Check sheet for the drawn part. Datum: minimum x, y, z corner. Units: mm. Give positions to 0.01 mm unless a question says otherwise; leave off trailing zeros. Write each loop counter-clockwise with the first axis right and the second up, starting at its lowest first coordinate (ties: lowest second). Pieces come first, ordered by that corner, then holes. Notation, with made-up numbers: (67, 24.25) - (109, 24.25) arc R19 ccw to (109, 44.25) - close; hole circle Ø2 at (55, 42). An arc over 180 degrees is marked (long way). Answer as a JSON object with one key per item and string values. Group by question number.
Item 1: Go/stop test with flat-tipped pins: pin 1 (6 mm diameter, centred on x = 109.07, z = 5.08, fed in from +Y); pin 2 (2 mm diameter, centred on x = 32.5, y = 6, fed in from +Z). Record where each tip stops, or that it passes through.
Item 2: Sectioned sample at A-A, the plane z = 5.08. Record the boundary of the cut face in (x, y).
Item 3: Scan lines: line 1 along X through (y, z) = (2, 5) (1 decimal); line 2 along Y through (x, z) = (50.5, 8.25); line 3 along Z through (x, y) = (7, 8.25). Record each from-to range of solid material in increasing order. Write a range as [from, to].
Item 4: Sectioned sample at B-B, the plane x = 39.5. Record the boundary of the cut face in (y, z), and give its area (3 significant figures).
Item 5: Sectioned sample at C-C, the plane y = 9.75. Record the boundary of the cut face in (x, z) (1 decimal).
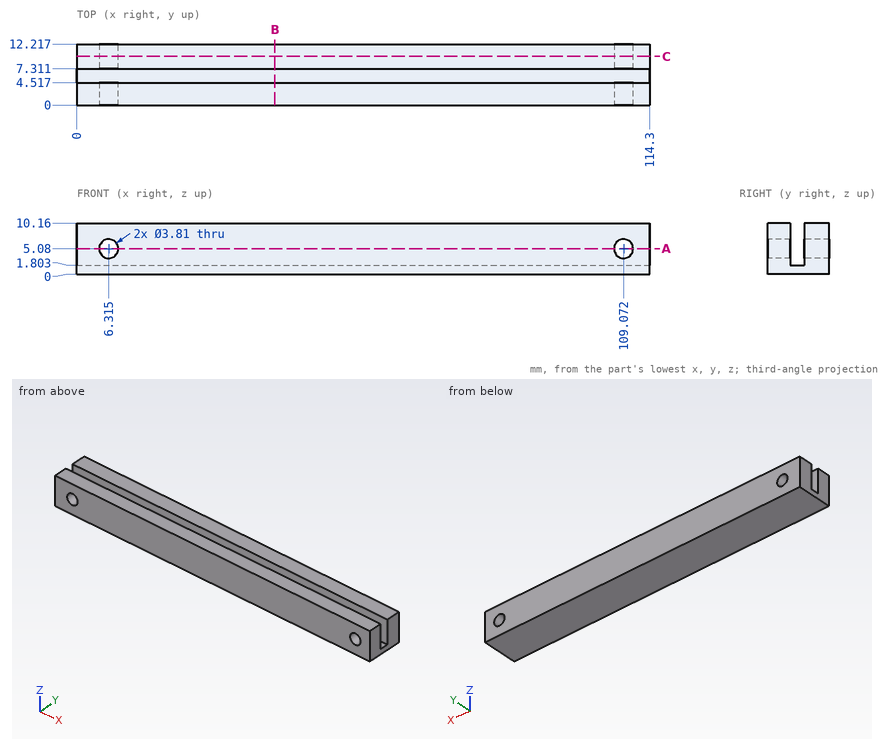
Geometry check:
{
 "1": {"pin 1": "y = 12.22", "pin 2": "z = 1.8"},
 "2": {"outline": "(0, 0) - (4.41, 0) - (4.41, 4.52) - (0, 4.52) - close; (0, 7.31) - (4.41, 7.31) - (4.41, 12.22) - (0, 12.22) - close; (8.22, 0) - (107.17, 0) - (107.17, 4.52) - (8.22, 4.52) - close; (8.22, 7.31) - (107.17, 7.31) - (107.17, 12.22) - (8.22, 12.22) - close; (110.98, 0) - (114.3, 0) - (114.3, 4.52) - (110.98, 4.52) - close; (110.98, 7.31) - (114.3, 7.31) - (114.3, 12.22) - (110.98, 12.22) - close"},
 "3": {"line 1": "[0, 4.4], [8.2, 107.2], [111, 114.3]", "line 2": "[0, 4.52], [7.31, 12.22]", "line 3": "[0, 3.3], [6.86, 10.16]"},
 "4": {"outline": "(0, 0) - (12.22, 0) - (12.22, 10.16) - (7.31, 10.16) - (7.31, 1.8) - (4.52, 1.8) - (4.52, 10.16) - (0, 10.16) - close", "area": "101 mm^2"},
 "5": {"outline": "(0, 0) - (114.3, 0) - (114.3, 10.2) - (0, 10.2) - close; hole circle Ø3.8 at (6.3, 5.1); hole circle Ø3.8 at (109.1, 5.1)"}
}
